```python
from build123d import *

# Parameters (mm, degrees)
SKETCH_1_R      = 10.5
SKETCH_1_R_2    = 5
SKETCH_1_R_3    = 1.5
EXTRUDE_1_DEPTH = 6


with BuildPart() as part:
    # Эскиз1 → Бобышка-Вытянуть1 (new body)
    with BuildSketch(Plane(origin=(0, 0, 0), x_dir=(1, 0, 0), z_dir=(0, 1, 0))):
        Polygon((-95, 14.235), (-15, 14.235), (-15, 20.235), (15, 20.235), (15, 14.235), (95, 14.235), (95, 7.5), (107, 7.5), (107, -7.5), (95, -7.5), (95, -14.235), (15, -14.235), (15, -20.235), (-15, -20.235), (-15, -14.235), (-95, -14.235), (-95, -7.5), (-107, -7.5), (-107, 7.5), (-95, 7.5), align=None)
        with Locations((-80, 0.265)):
            Circle(SKETCH_1_R, mode=Mode.SUBTRACT)
        with Locations((80, 0.265)):
            Circle(SKETCH_1_R, mode=Mode.SUBTRACT)
        with Locations((0, 0.265)):
            Circle(SKETCH_1_R_2, mode=Mode.SUBTRACT)
        with Locations((-5.656854249, 5.921854249)):
            Circle(SKETCH_1_R_3, mode=Mode.SUBTRACT)
        with Locations((5.656854249, 5.921854249)):
            Circle(SKETCH_1_R_3, mode=Mode.SUBTRACT)
        with Locations((5.656854249, -5.391854249)):
            Circle(SKETCH_1_R_3, mode=Mode.SUBTRACT)
        with Locations((-5.656854249, -5.391854249)):
            Circle(SKETCH_1_R_3, mode=Mode.SUBTRACT)
    extrude(amount=EXTRUDE_1_DEPTH)


solid = part.part
```
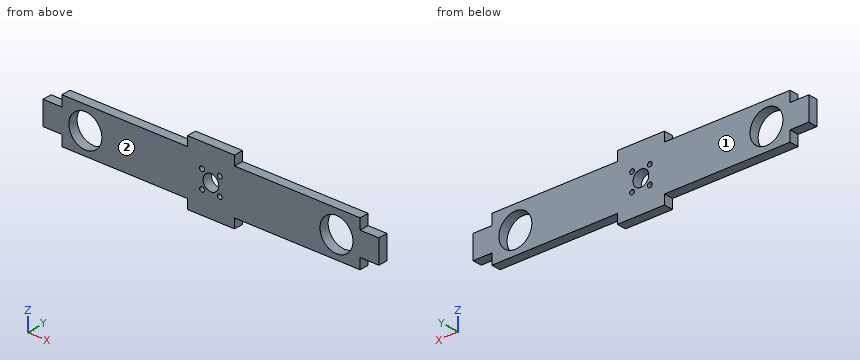
Can you work these out from the model? Positions are in its coordinate system, mm. Face numbers are marked on the shaded views. Coordinates: 2 decimals unless noted, no trailing zeros. Loops run counter-clockwise (first coordinate to the right, second up) from the corner with the lowest first, then second, coordinate; pieces in that order, holes last. Notation, with made-up numbers: (51.25, 79.25) -> (68.25, 79.25) arc R29 ccw to (68.25, 99.25) -> close; hole circle Ø3 at (49.25, 32.5). An arc over 180 degrees is marked (long way). Put each result on its own line as item: value. Start each with the question number.
Q1. If I drill on line 1 (Z direction, x = 80, y = 2.05) (3 decimals); line 2 (X direction, y = 2.4, z = -6); line 3 (X direction, y = 3.75, z = -9), over which ranges is the centre line in solid material (lowest first)? Write a range as [from, to].
Q2. I want a section at D-D (y = 0.9). Write out the boundary of the cut face in (x, z) (3 decimals).
Q3. I want a section at A-A (x = -80). Write out the boundary of the cut face in (y, z) (3 decimals), plus the area to 3 significant figures.
Q4. I'm going to push flat-ended pins straight in: P1, Ø6, axis at x = 0, z = -0.265, coming from the -Y side; P2, Ø12, axis at x = 0, z = 8.5, coming from the -Y side; P3, Ø3, axis at y = 2, z = -16.5, coming from the -X side; P4, Ø3, axis at y = 3, z = -10.5, coming from the +X side. Where does each tip first touch, or does it pass through?
Q5. I want a section at C-C (x = 0). Write out the boundary of the cut face in (y, z) (3 decimals).
Q6. Thinking about a two-plate mould opening in Y: for the marked faces 1 and 2, which applies, pulls with the +Y half, pulls with the -Y half, needs draft (parallel to the pull), parting line crosses it, or undercut?
Q7. I want a section at B-B (z = 1.5). Write out the boundary of the cut face in (x, y), plus the area to 3 significant figures.
Taken from the geometry:
1. line 1: z = [-14.235, -10.765], [10.235, 14.235]
1. line 2: x = [-107, -88.8], [-71.2, -7.15], [-4.16, 4.16], [7.15, 71.2], [88.8, 107]
1. line 3: x = [-95, -85.83], [-74.17, 74.17], [85.83, 95]
2. outline: (-107, -7.5) -> (-95, -7.5) -> (-95, -14.235) -> (-15, -14.235) -> (-15, -20.235) -> (15, -20.235) -> (15, -14.235) -> (95, -14.235) -> (95, -7.5) -> (107, -7.5) -> (107, 7.5) -> (95, 7.5) -> (95, 14.235) -> (15, 14.235) -> (15, 20.235) -> (-15, 20.235) -> (-15, 14.235) -> (-95, 14.235) -> (-95, 7.5) -> (-107, 7.5) -> close; hole circle Ø21 at (-80, -0.265); hole circle Ø3 at (-5.657, -5.922); hole circle Ø3 at (-5.657, 5.392); hole circle Ø10 at (0, -0.265); hole circle Ø3 at (5.657, -5.922); hole circle Ø3 at (5.657, 5.392); hole circle Ø21 at (80, -0.265)
3. outline: (0, -14.235) -> (6, -14.235) -> (6, -10.765) -> (0, -10.765) -> close; (0, 10.235) -> (6, 10.235) -> (6, 14.235) -> (0, 14.235) -> close
3. area: 44.8 mm2
4. P1: passes through
4. P2: stops at y = 0
4. P3: stops at x = -15
4. P4: stops at x = 95
5. outline: (0, -20.235) -> (6, -20.235) -> (6, -5.265) -> (0, -5.265) -> close; (0, 4.735) -> (6, 4.735) -> (6, 20.235) -> (0, 20.235) -> close
6. face 1: pulls with the +Y half
6. face 2: pulls with the -Y half
7. outline: (-107, 0) -> (-90.35, 0) -> (-90.35, 6) -> (-107, 6) -> close; (-69.65, 0) -> (-4.68, 0) -> (-4.68, 6) -> (-69.65, 6) -> close; (4.68, 0) -> (69.65, 0) -> (69.65, 6) -> (4.68, 6) -> close; (90.35, 0) -> (107, 0) -> (107, 6) -> (90.35, 6) -> close
7. area: 979 mm2
